from build123d import *

# Parameters (mm, degrees)
EXTRUDE_1_DEPTH = 18.7
SKETCH_2_R      = 0.75
EXTRUDE_2_DEPTH = 11.3


with BuildPart() as part:
    # 草图1 → 凸台-拉伸1 (new body)
    with BuildSketch(Plane(origin=(0, 0, 0), x_dir=(1, 0, 0), z_dir=(0, 1, 0))):
        with BuildLine():
            Line((4.808326112, 5.95), (-4.808326112, 5.95))
            ThreePointArc((-4.808326112, 5.95), (-7.65, 0), (-4.808326112, -5.95))
            Line((-4.808326112, -5.95), (4.808326112, -5.95))
            ThreePointArc((4.808326112, -5.95), (7.65, 0), (4.808326112, 5.95))
        make_face()
    extrude(amount=EXTRUDE_1_DEPTH)

    # 草图2 → 凸台-拉伸2 (add)
    with BuildSketch(Plane(origin=(0, 18.7, 0), x_dir=(1, 0, 0), z_dir=(0, 1, 0))):
        with Locations(Location((0, 0, 0), (0, 0, 270))):
            Circle(SKETCH_2_R)
    extrude(amount=EXTRUDE_2_DEPTH)


solid = part.part
Input: part model. Units: mm. Frame: model coordinates. A direction names the side the tool comes from. Round coordinates to 2 decimals unless told otherwise and drop trailing zeros. Write each loop counter-clockwise with the first axis right and the second up, starting at its lowest first coordinate (ties: lowest second). Pieces come first, ordered by that corner, then holes.
1) Ray query, L1, parallel to Y at x = 2.5, z = -1; L2, parallel to X at y = 11.75, z = -0.25; L3, parallel to Z at x = 5.25, y = 6. Return the intervals inside material, ascending.
2) Cut plane D-D (y = 23.5). Return the cut outline in (x, z).
3) Cut plane C-C (y = 17.5). Return the cut outline in (x, z), then the cut area to 3 significant figures.
4) Contact query for flat-ended pins moving along their axis: P1, Ø4, axis at x = -5.5, z = 1, coming from the +Y side; P2, Ø6, axis at y = 12, z = 4.5, coming from the -X side; P3, Ø1, axis at y = 18.5, z = -3.5, coming from the -X side. Output: stop coordinate, or through.
5) Reachability of faces 1 (the flat face through (0, 0, 0)), 2 (the cylindrical face through (0.225, 24.271, 0.715)) from +Z, -Z, +X, -X, +Y, -Y: full face, straight path, thin tool, end or side. Return the list, or none.
6) Cut plane A-A (z = 0). Return the cut outline in (x, y), then the cut area to 3 significant figures.
7) Cut plane B-B (x = 0). Return the cut outline in (y, z).
Geometry says:
1. L1: y = 0 to 18.7
1. L2: x = -7.65 to 7.65
1. L3: z = -5.56 to 5.56
2. outline: circle Ø1.5 at (0, 0)
3. outline: (-4.81, -5.95) - (4.81, -5.95) arc R7.65 ccw to (4.81, 5.95) - (-4.81, 5.95) arc R7.65 ccw to start
3. area: 162 mm2
4. P1: stops at y = 18.7
4. P2: stops at x = -7.5
4. P3: stops at x = -7.04
5. face 1: +Z, -Z, +X, -X, -Y
5. face 2: +Y
6. outline: (-7.65, 0) - (7.65, 0) - (7.65, 18.7) - (0.75, 18.7) - (0.75, 30) - (-0.75, 30) - (-0.75, 18.7) - (-7.65, 18.7) - close
6. area: 303 mm2
7. outline: (0, -5.95) - (18.7, -5.95) - (18.7, -0.75) - (30, -0.75) - (30, 0.75) - (18.7, 0.75) - (18.7, 5.95) - (0, 5.95) - close
